```python
from build123d import *

# Parameters (mm, degrees)
SKETCH_1_W          = 65
SKETCH_1_H          = 40
SKETCH_1_R          = 1.65
SKETCH_1_R_2        = 5.2
EXTRUDE_1_DEPTH     = 3
SKETCH_2_R          = 1.5
CUT_EXTRUDE_1_DEPTH = 3
SKETCH_3_W          = 65
SKETCH_3_H          = 5
CUT_EXTRUDE_2_DEPTH = 10
SKETCH_4_W          = 65
SKETCH_4_H          = 5
CUT_EXTRUDE_3_DEPTH = 10
FILLET_2_R          = 3


with BuildPart() as part:
    # 草图1 → 凸台-拉伸1 (new body)
    with BuildSketch(Plane.XY):
        Rectangle(SKETCH_1_W, SKETCH_1_H)
        with Locations((-5.656854249, 5.656854249)):
            Circle(SKETCH_1_R, mode=Mode.SUBTRACT)
        Circle(SKETCH_1_R_2, mode=Mode.SUBTRACT)
        with Locations((5.656854249, 5.656854249)):
            Circle(SKETCH_1_R, mode=Mode.SUBTRACT)
        with Locations((5.656854249, -5.656854249)):
            Circle(SKETCH_1_R, mode=Mode.SUBTRACT)
        with Locations((-5.656854249, -5.656854249)):
            Circle(SKETCH_1_R, mode=Mode.SUBTRACT)
    extrude(amount=EXTRUDE_1_DEPTH)

    # 草图2 → 切除-拉伸1 (cut)
    with BuildSketch(Plane.XY.offset(3)):
        with Locations((29.5, 10)):
            Circle(SKETCH_2_R)
        with Locations((29.5, -10)):
            Circle(SKETCH_2_R)
        with Locations((-29.5, -10)):
            Circle(SKETCH_2_R)
        with Locations((-29.5, 10)):
            Circle(SKETCH_2_R)
    extrude(amount=-CUT_EXTRUDE_1_DEPTH, mode=Mode.SUBTRACT)

    # 草图3 → 切除-拉伸2 (cut)
    with BuildSketch(Plane(origin=(0, 0, 0), x_dir=(-1, 0, 0), z_dir=(0, 0, -1))):
        with Locations((0, 17.5)):
            Rectangle(SKETCH_3_W, SKETCH_3_H)
    extrude(amount=-CUT_EXTRUDE_2_DEPTH, mode=Mode.SUBTRACT)

    # 草图4 → 切除-拉伸3 (cut)
    with BuildSketch(Plane.XY.offset(3)):
        with Locations((0, -17.5)):
            Rectangle(SKETCH_4_W, SKETCH_4_H)
    extrude(amount=-CUT_EXTRUDE_3_DEPTH, mode=Mode.SUBTRACT)

    # 圆角2
    fillet_2_edges = [part.edges().sort_by_distance(p)[0] for p in [
        (-32.5, 15, 1.5),
        (32.5, 15, 1.5),
        (-32.5, -15, 1.5),
        (32.5, -15, 1.5),
    ]]
    fillet(fillet_2_edges, radius=FILLET_2_R)


solid = part.part
```
Geometry check sheet. Reference: the model listing, model coordinates, mm. Give positions to 0.01 mm unless a question says otherwise; leave off trailing zeros. Write each loop counter-clockwise with the first axis right and the second up, starting at its lowest first coordinate (ties: lowest second). Pieces come first, ordered by that corner, then holes. Notation, with made-up numbers: (-18.5, 23) - (11.5, 23) arc R8 ccw to (11.5, 33) - close; hole circle Ø9 at (-36.5, -21). An arc over 180 degrees is marked (long way). Use a Markdown table: item, result.
Q1. Go/stop test with a flat-tipped pin: P1, Ø2.5, axis at x = 29.5, y = -10, coming from the -Z side. Record where the tip stops, or that it passes through.
Computed:
| item | result |
|---|---|
| P1 | passes through |
Q2. Draft check along Y on faces 1 (the face through (-0.677, 5.156, 1.479)), 2 (the face through (0, 7, 0)), 3 (the face through (31.6, -14.14, 1.48)). Enter one of: pulls with the +Y half, pulls with the -Y half, needs draft (parallel to the pull), parting line crosses it, or undercut.
Computed:
| item | result |
|---|---|
| face 1 | undercut |
| face 2 | needs draft |
| face 3 | pulls with the -Y half |
Q3. Section check B-B, the plane y = -10. Enter the section's corners in (x, z), then the cut area to 3 significant figures.
Computed:
| item | result |
|---|---|
| outline | (-32.5, 0) - (-31, 0) - (-31, 3) - (-32.5, 3) - close; (-28, 0) - (28, 0) - (28, 3) - (-28, 3) - close; (31, 0) - (32.5, 0) - (32.5, 3) - (31, 3) - close |
| area | 177 mm² |
Q4. Section check D-D, the plane y = 1.5. Enter the section's corners in (x, z).
Computed:
| item | result |
|---|---|
| outline | (-32.5, 0) - (-4.98, 0) - (-4.98, 3) - (-32.5, 3) - close; (4.98, 0) - (32.5, 0) - (32.5, 3) - (4.98, 3) - close |
Q5. Thickness scan on L1, parallel to Y at x = 29.5, z = 1.8; L2, parallel to X at y = -10.25, z = 1.45; L3, parallel to Y at x = 0, z = 1.1. Record the ranges inside material, lowest first. Write a range as [from, to].
Computed:
| item | result |
|---|---|
| L1 | y = [-15, -11.5], [-8.5, 8.5], [11.5, 15] |
| L2 | x = [-32.5, -30.98], [-28.02, 28.02], [30.98, 32.5] |
| L3 | y = [-15, -5.2], [5.2, 15] |
Q6. Section check A-A, the plane x = 0. Enter the section's corners in (y, z).
Computed:
| item | result |
|---|---|
| outline | (-15, 0) - (-5.2, 0) - (-5.2, 3) - (-15, 3) - close; (5.2, 0) - (15, 0) - (15, 3) - (5.2, 3) - close |
Q7. Section check C-C, the plane z = 1.75. Give the number of separate pieces and of enclosed holes in the cut face, then the cut area to 3 significant figures.
Computed:
| item | result |
|---|---|
| separate pieces | 1 |
| enclosed holes | 9 |
| area | 1,790 mm² |
